The model under review builds one solid part; all positions refer to its coordinate system, in mm. Coordinates: 2 decimals unless noted, no trailing zeros. Loops run counter-clockwise (first coordinate to the right, second up) from the corner with the lowest first, then second, coordinate; pieces in that order, holes last. Notation, with made-up numbers: M 73.5,57.5 L 130.5,57.5 A16 cw 130.5,76.5 Z; hole C 2,-17.75 d6. An arc over 180 degrees is marked long. One line per item, written item: value.
Autodesk Inventor part; units mm, degrees
ref_plane "Start Plane" through (0, 0, -6.1539) normal (0, 0, 1) x (1, 0, 0)
ref_plane "End Plane" through (0, 0, 227.4965) normal (0, 0, 1) x (1, 0, 0)
ref_plane "Work Plane4" through (-10.4438, -2.1758, 233.1995) normal (0.7278, 0.1516, 0.6689) x (0.6826, -0.0661, -0.7278)
ref_plane "Start Plane" through (0, 0, -6.1539) normal (0, 0, 1) x (1, 0, 0)
ref_plane "End Plane" through (0, 0, 227.4965) normal (0, 0, 1) x (1, 0, 0)
sketch "Sketch" plane through (0, 0, 0) normal (0, 0, 1) x (1, 0, 0)
  circle A0 centre (0, 0) radius 6.9342
  circle A1 centre (0, 0) radius 10.668
  dimension "d0" = 21.336
  dimension "d1" = 3.7338
extrude "Body" add sketch "Sketch" along normal up to surface (233.6505 mm away) from surface at -6.1539
sketch "Sketch3" plane through (0, 0, 0) normal (0, 0, 1) x (1, 0, 0)
  line L0 (0, 0) -> (10, 0)
ref_plane "Work Plane3" through (0, 0, 0) normal (0, -1, 0) x (1, 0, 0)
sketch "Sketch4" plane through (0, 0, 0) normal (0, -1, 0) x (1, 0, 0)
  line L0 (-2, -6.1539) -> (12, -6.1539)
  line L1 (-2, 227.4965) -> (12, 227.4965)
  dimension "d7" = 233.6505
ref_plane "Work Plane4" through (-10.4438, -2.1758, 233.1995) normal (0.7278, 0.1516, 0.6689) x (0.6826, -0.0661, -0.7278)
split "Split1" plane through (-10.4438, -2.1758, 233.1995) removes the side toward (0.7278, 0.1516, 0.6689)
ref_plane "Work Plane5" through (-2.0318, -10.4727, 227.5652) normal (0.096, 0.4946, 0.8638) x (0.9951, -0.0255, -0.096)
split "Split2" plane through (-2.0318, -10.4727, 227.5652) removes the side toward (0.096, 0.4946, 0.8638)
ref_plane "Work Plane6" through (6.5371, -8.4304, 233.0164) normal (-0.4523, 0.5834, 0.6746) x (0.8778, 0.1576, 0.4523)
split "Split3" plane through (6.5371, -8.4304, 233.0164) removes the side toward (-0.4523, 0.5834, 0.6746)
ref_plane "Work Plane7" through (-2.0318, -10.4727, -6.2226) normal (0.096, 0.4946, -0.8638) x (0.9324, -0.3485, -0.096)
split "Split4" plane through (-2.0318, -10.4727, -6.2226) removes the side toward (0.096, 0.4946, -0.8638)
ref_plane "Work Plane8" through (-10.4438, -2.1758, -11.8569) normal (0.7278, 0.1516, -0.6689) x (-0.5994, -0.3332, -0.7278)
split "Split5" plane through (-10.4438, -2.1758, -11.8569) removes the side toward (0.7278, 0.1516, -0.6689)
ref_plane "Work Plane9" through (6.5371, -8.4304, -11.6738) normal (-0.4523, 0.5834, -0.6746) x (0.3712, 0.8109, 0.4523)
split "Split6" plane through (6.5371, -8.4304, -11.6738) removes the side toward (-0.4523, 0.5834, -0.6746)
equation "\"d0\" = G_H"
equation "\"d1\" = G_T"
equation "\"d2\" = G_L"
equation "\"G_H\" = 21.336"
equation "\"G_T\" = 3.7338"
equation "\"G_L\" = 233.65046"
equation "\"G_OFFSET_START\" = 6.15394"
equation "\"G_OFFSET_END\" = 6.15394"
equation "\"d4\" = -G_OFFSET_START"
equation "\"d5\" = G_OFFSET_END + B_L"
equation "\"B_L\" = 221.34258"
properties part number "ANSI - 1/2 x 0.147 - 9.199" material "Steel, Mild"
(1) Add section B-B on x = 0. State the section outline as (y, z) points.
Checks:
outline: M -10.67,-2.42 L -6.93,-1.57 L -6.93,222.91 L -10.67,223.76 Z; M 6.93,6 L 10.67,9.23 L 10.67,212.12 L 6.93,215.35 Z
(2) Draft analysis for pull direction X (two halves, no side actions). For faces 1 (the face through (-1.389, -10.577, 109.036)), 2 (the face through (-0.903, -6.875, 109.066)), 3 (the face through (-6.794, 3.292, 213.94)), state which applies: pulls with the +X half, pulls with the -X half, needs draft (parallel to the pull), parting line crosses it, or undercut.
Checks:
face 1: parting line crosses it
face 2: undercut
face 3: pulls with the -X half
(3) To check wall thickness, follow L1, parallel to X at y = -0.5, z = 30.5; L2, parallel to Y at x = 0, z = 100; L3, parallel to Y at x = 6.25, z = 53. State the ranges of each line that lie inside material, in increasing order. Write a range as [from, to].
Checks:
L1: [-10.66, -6.92], [6.92, 10.66]
L2: [-10.67, -6.93], [6.93, 10.67]
L3: [-8.65, -3], [3, 8.65]
(4) Add section A-A on y = -3.5. State the section outline as (x, z) points.
Checks:
outline: M -10.08,3.73 L -5.99,0.99 L -5.99,220.36 L -10.08,217.61 Z; M 5.99,5.72 L 10.08,10.17 L 10.08,211.17 L 5.99,215.62 Z
(5) Add section C-C on z = 98. State the section outline as (x, y) points, then the cut area to 3 significant figures.
Checks:
outline: C 0,0 d21.34; hole C 0,0 d13.87
area: 206 mm^2
(6) Insertion check: pin 1 Ø1 at (x, y) = (7, 3) entering from -Z; pin 2 Ø2 at (y, z) = (-6.5, 21) entering from -X; pin 3 Ø6 at (y, z) = (5.5, 152) entering from +X; pin 4 Ø8.5 at (x, y) = (0, 0) entering from +Z. Each pin has a flat end and moves straight along its axis. Give the tip position at first contact, or say it passes through.
Checks:
pin 1: z = 7.74
pin 2: x = -9.14
pin 3: x = 10.37
pin 4: through
